Model file for the job. Use its own axes, mm. Face numbers are marked on the shaded views. A direction names the side the tool comes from. Coordinates: 2 decimals unless noted, no trailing zeros. Order: outer loops, then holes, each group sorted by start corner. A loop starts at its lowest first (then second) coordinate and runs counter-clockwise, first axis right, second up. Notation, with made-up numbers: (-3.5, 66.25) -> (35.5, 66.25) arc R19 ccw to (35.5, 79.25) -> close; hole circle Ø11 at (30.5, -5). An arc over 180 degrees is marked (long way). Use CSV: the item, a comma, the result in double quotes. Start each with the question number.
(1) Cut at B-B on x = -18.6. Write the cut outline in (y, z).
(2) Cut at D-D on z = 0. Give the number of separate pieces and of enclosed holes in the cut face, plus the area to 3 significant figures.
(3) Cut at C-C on y = 14.53. Write the cut outline in (x, z).
(4) Probe L1, parallel to X at y = 1.25, z = 0; L2, parallel to Z at x = 0, y = 0.7; L3, parallel to X at y = 13, z = -9.75. List the from-to ranges inside material, lowest first.
(5) Cut at A-A on y = 28. Write the cut outline in (x, z), plus the area to 3 significant figures.
(6) Pull direction X, two halves, no side cores. Call the marked faces 1, 2 and 3: pulls with the +X half, pulls with the -X half, needs draft (parallel to the pull), parting line crosses it, or undercut.
(7) Tool access for the marked faces 4 and 5: list every direction of +Z, -Z, +X, -X, +Y, -Y with a clear straight run to the whole face (end or side of a thin tool).
(8) Pin check, flat tips, straight feed: pin 1 Ø2.5 at (y, z) = (14.53, 0) entering from +X; pin 2 Ø10.5 at (x, z) = (0, 0) entering from +Y. Stop position of each tip, or through.
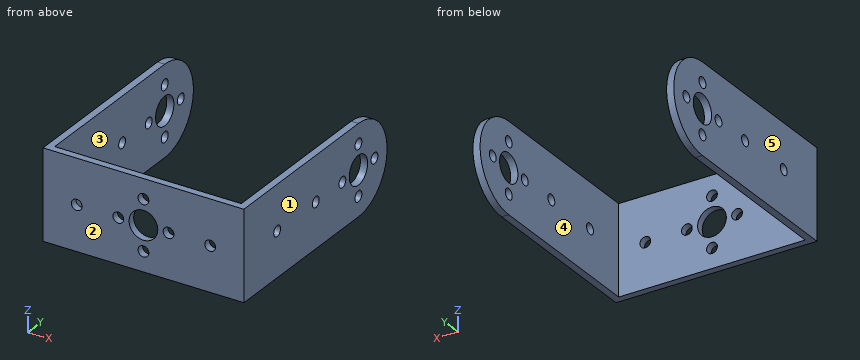
```python
from build123d import *

# Parameters (mm, degrees)
SKETCH1_W           = 52
SKETCH1_H           = 25
SKETCH1_R           = 4
SKETCH1_R_2         = 1.5
BOSS_EXTRUDE1_DEPTH = 2
SKETCH3_R           = 4
SKETCH3_R_2         = 1.5
BOSS_EXTRUDE2_DEPTH = 2
SKETCH4_R           = 4
SKETCH4_R_2         = 1.5
BOSS_EXTRUDE3_DEPTH = 2


with BuildPart() as part:
    # Sketch1 → Boss-Extrude1 (new body)
    with BuildSketch(Plane(origin=(0, 0, 0), x_dir=(1, 0, 0), z_dir=(0, 1, 0))):
        Rectangle(SKETCH1_W, SKETCH1_H)
        Circle(SKETCH1_R, mode=Mode.SUBTRACT)
        with Locations((18.6, 0)):
            Circle(SKETCH1_R_2, mode=Mode.SUBTRACT)
        with Locations((0, 7)):
            Circle(SKETCH1_R_2, mode=Mode.SUBTRACT)
        with Locations((7, 0)):
            Circle(SKETCH1_R_2, mode=Mode.SUBTRACT)
        with Locations((0, -7)):
            Circle(SKETCH1_R_2, mode=Mode.SUBTRACT)
        with Locations((-7, 0)):
            Circle(SKETCH1_R_2, mode=Mode.SUBTRACT)
        with Locations((-18.6, 0)):
            Circle(SKETCH1_R_2, mode=Mode.SUBTRACT)
    extrude(amount=BOSS_EXTRUDE1_DEPTH)

    # Sketch3 → Boss-Extrude2 (add)
    with BuildSketch(Plane(origin=(26, 0, 0), x_dir=(0, 0, -1), z_dir=(1, 0, 0))):
        with BuildLine():
            Line((-12.5, 0), (12.5, 0))
            Line((12.5, 0), (12.5, 50))
            ThreePointArc((12.5, 50), (0, 62.5), (-12.5, 50))
            Line((-12.5, 50), (-12.5, 0))
        make_face()
        with Locations((0, 50)):
            Circle(SKETCH3_R, mode=Mode.SUBTRACT)
        with Locations((0, 43)):
            Circle(SKETCH3_R_2, mode=Mode.SUBTRACT)
        with Locations((7, 50)):
            Circle(SKETCH3_R_2, mode=Mode.SUBTRACT)
        with Locations((0, 57)):
            Circle(SKETCH3_R_2, mode=Mode.SUBTRACT)
        with Locations((-7, 50)):
            Circle(SKETCH3_R_2, mode=Mode.SUBTRACT)
        with Locations((0, 31.4)):
            Circle(SKETCH3_R_2, mode=Mode.SUBTRACT)
        with Locations((0, 14.53)):
            Circle(SKETCH3_R_2, mode=Mode.SUBTRACT)
    extrude(amount=BOSS_EXTRUDE2_DEPTH)

    # Sketch4 → Boss-Extrude3 (add)
    with BuildSketch(Plane.ZY.offset(26)):
        with BuildLine():
            Line((-12.5, 0), (12.5, 0))
            Line((12.5, 0), (12.5, 50))
            ThreePointArc((12.5, 50), (0, 62.5), (-12.5, 50))
            Line((-12.5, 50), (-12.5, 0))
        make_face()
        with Locations((0, 50)):
            Circle(SKETCH4_R, mode=Mode.SUBTRACT)
        with Locations((0, 57)):
            Circle(SKETCH4_R_2, mode=Mode.SUBTRACT)
        with Locations((7, 50)):
            Circle(SKETCH4_R_2, mode=Mode.SUBTRACT)
        with Locations((-7, 50)):
            Circle(SKETCH4_R_2, mode=Mode.SUBTRACT)
        with Locations((0, 43)):
            Circle(SKETCH4_R_2, mode=Mode.SUBTRACT)
        with Locations((0, 31.4)):
            Circle(SKETCH4_R_2, mode=Mode.SUBTRACT)
        with Locations((0, 14.53)):
            Circle(SKETCH4_R_2, mode=Mode.SUBTRACT)
    extrude(amount=BOSS_EXTRUDE3_DEPTH)


solid = part.part
```
Outcome:
1,outline,"(0, -12.5) -> (2, -12.5) -> (2, -1.5) -> (0, -1.5) -> close; (0, 1.5) -> (2, 1.5) -> (2, 12.5) -> (0, 12.5) -> close"
2,separate pieces,"16"
2,enclosed holes,"0"
2,area,"234 mm2"
3,outline,"(-28, -12.5) -> (-26, -12.5) -> (-26, -1.5) -> (-28, -1.5) -> close; (-28, 1.5) -> (-26, 1.5) -> (-26, 12.5) -> (-28, 12.5) -> close; (26, -12.5) -> (28, -12.5) -> (28, -1.5) -> (26, -1.5) -> close; (26, 1.5) -> (28, 1.5) -> (28, 12.5) -> (26, 12.5) -> close"
4,L1,"-28 to -20.1, -17.1 to -8.5, -5.5 to -4, 4 to 5.5, 8.5 to 17.1, 20.1 to 28"
4,L2,"-12.5 to -8.5, -5.5 to -4, 4 to 5.5, 8.5 to 12.5"
4,L3,"-28 to -26, 26 to 28"
5,outline,"(-28, -12.5) -> (-26, -12.5) -> (-26, 12.5) -> (-28, 12.5) -> close; (26, -12.5) -> (28, -12.5) -> (28, 12.5) -> (26, 12.5) -> close"
5,area,"100 mm2"
6,face 1,"pulls with the +X half"
6,face 2,"needs draft"
6,face 3,"undercut"
7,face 4,"+Z, -Z, +Y"
7,face 5,"+Z, -Z, -X, +Y, -Y"
8,pin 1,"through"
8,pin 2,"y = 2"
